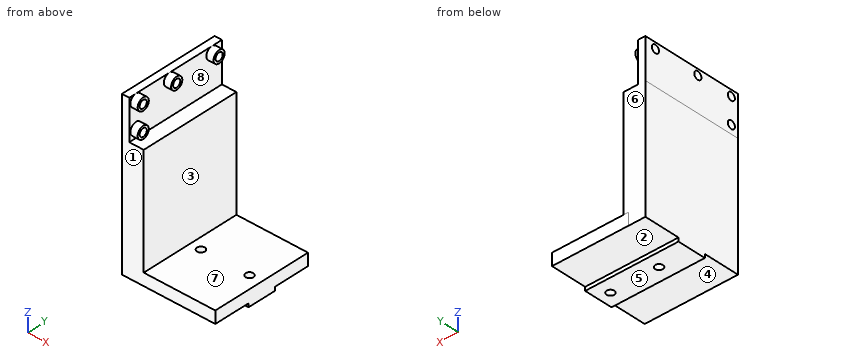
```python
from build123d import *

# Parameters (mm, degrees)
SKETCH1_W               = 31.5
SKETCH1_H               = 41.5
BOSS_EXTRUDE1_DEPTH     = 5
SKETCH3_W               = 6
SKETCH3_H               = 41.48411863
BOSS_EXTRUDE3_DEPTH     = 50.5
SKETCH5_W               = 3
SKETCH5_H               = 41.48411863
BOSS_EXTRUDE4_DEPTH     = 16.5
SKETCH6_W               = 50.5
SKETCH6_H               = 41.48411863
BOSS_EXTRUDE6_DEPTH     = 2
SKETCH4_R               = 2.5
SKETCH4_R_2             = 1.6
BOSS_EXTRUDE7_DEPTH     = 3
SKETCH4_6_R             = 1.6
CUT_EXTRUDE1_DEPTH      = 4
CUT_EXTRUDE1_DEPTH_BACK = 36.459931403
SKETCH7_W               = 1.5
SKETCH7_H               = 11.8
BOSS_EXTRUDE8_DEPTH     = 37.5
SKETCH8_R               = 1.6
CUT_EXTRUDE2_DEPTH      = 7.5
BOSS_EXTRUDE9_DEPTH     = 0.959931


with BuildPart() as part:
    # Sketch1 → Boss-Extrude1 (new body)
    with BuildSketch(Plane.XY):
        with Locations((-107.290068597, -86.48411863)):
            Rectangle(SKETCH1_W, SKETCH1_H)
    extrude(amount=BOSS_EXTRUDE1_DEPTH)

    # Sketch3 → Boss-Extrude3 (add)
    with BuildSketch(Plane.XY):
        with Locations((-126.040068597, -86.492059315)):
            Rectangle(SKETCH3_W, SKETCH3_H)
    extrude(amount=BOSS_EXTRUDE3_DEPTH)

    # Sketch5 → Boss-Extrude4 (add)
    with BuildSketch(Plane.XY.offset(50.5)):
        with Locations((-128.5, -86.492059315)):
            Rectangle(SKETCH5_W, SKETCH5_H)
    extrude(amount=BOSS_EXTRUDE4_DEPTH)

    # Sketch6 → Boss-Extrude6 (add)
    with BuildSketch(Plane(origin=(-123.040068597, 0, 0), x_dir=(0, 0, -1), z_dir=(1, 0, 0))):
        with Locations((-25.25, -86.492059315)):
            Rectangle(SKETCH6_W, SKETCH6_H)
    extrude(amount=BOSS_EXTRUDE6_DEPTH)

    # Sketch4 → Boss-Extrude7 (add)
    with BuildSketch(Plane.ZY.offset(127)):
        with Locations((54, -104.25)):
            Circle(SKETCH4_R)
        with Locations((54, -104.25)):
            Circle(SKETCH4_R_2, mode=Mode.SUBTRACT)
        with Locations((64.5, -104.25)):
            Circle(SKETCH4_R)
        with Locations((64.5, -104.25)):
            Circle(SKETCH4_R_2, mode=Mode.SUBTRACT)
        with Locations((64.5, -89.25)):
            Circle(SKETCH4_R)
        with Locations((64.5, -89.25)):
            Circle(SKETCH4_R_2, mode=Mode.SUBTRACT)
        with Locations((64.5, -70.25)):
            Circle(SKETCH4_R)
        with Locations((64.5, -70.25)):
            Circle(SKETCH4_R_2, mode=Mode.SUBTRACT)
    extrude(amount=-BOSS_EXTRUDE7_DEPTH)

    # Sketch4<6> → Cut-Extrude1 (cut, two sides)
    with BuildSketch(Plane.ZY.offset(127)) as cut_extrude1_sk:
        with Locations((64.5, -104.25)):
            Circle(SKETCH4_6_R)
        with Locations((64.5, -89.25)):
            Circle(SKETCH4_6_R)
        with Locations((64.5, -70.25)):
            Circle(SKETCH4_6_R)
        with Locations((54, -104.25)):
            Circle(SKETCH4_6_R)
    extrude(amount=CUT_EXTRUDE1_DEPTH, mode=Mode.SUBTRACT)
    extrude(cut_extrude1_sk.sketch, amount=-CUT_EXTRUDE1_DEPTH_BACK, mode=Mode.SUBTRACT)

    # Sketch7 → Boss-Extrude8 (add)
    with BuildSketch(Plane(origin=(-91.540068597, 0, 0), x_dir=(0, 0, -1), z_dir=(1, 0, 0))):
        with Locations((0.75, -86.48411863)):
            Rectangle(SKETCH7_W, SKETCH7_H)
    extrude(amount=-BOSS_EXTRUDE8_DEPTH)

    # Sketch8 → Cut-Extrude2 (cut, through all)
    with BuildSketch(Plane.XY.offset(5)):
        with Locations((-116.540068597, -86.490848024)):
            Circle(SKETCH8_R)
        with Locations((-96.540068597, -86.485464509)):
            Circle(SKETCH8_R)
    extrude(amount=-CUT_EXTRUDE2_DEPTH, mode=Mode.SUBTRACT)

    # Sketch9 → Boss-Extrude9 (add)
    with BuildSketch(Plane.ZY.offset(129.040068597)):
        Polygon((50.5, -65.75), (0, -65.75), (0, -80.58411863), (-1.5, -80.58411863), (-1.5, -92.38411863), (0, -92.38411863), (0, -107.23411863), (50.5, -107.23411863), align=None)
    extrude(amount=BOSS_EXTRUDE9_DEPTH)


solid = part.part
```
Check sheet for the modelled part. Datum: model origin and axes. Units: mm. Face numbers are marked on the shaded views. A direction names the side the tool comes from. Coordinates: 2 decimals unless noted, no trailing zeros. Loops run counter-clockwise (first coordinate to the right, second up) from the corner with the lowest first, then second, coordinate; pieces in that order, holes last. Notation, with made-up numbers: M 32,-7 L 78,-7 A12 ccw 78,14 Z; hole C 71.25,78.25 d9. An arc over 180 degrees is marked long. Answer as a JSON object with one key per item and string values.
1. Scan lines: L1, parallel to Z at x = -128.45, y = -104.25; L2, parallel to Z at x = -113, y = -97.5; L3, parallel to X at y = -69.5, z = 29.5. Record each from-to range of solid material in increasing order. Write a range as from..to.
Outcome:
{"L1": "0..52.4, 55.6..62.9, 66.1..67", "L2": "0..5", "L3": "-130..-121.04"}
2. Sectioned sample at C-C on z = 54. Record the cut outline in (x, y).
Outcome:
{"outline": "M -130,-107.23 L -127,-107.23 L -127,-106.75 L -124,-106.75 L -124,-105.85 L -130,-105.85 Z; M -130,-102.65 L -124,-102.65 L -124,-101.75 L -127,-101.75 L -127,-65.75 L -130,-65.75 Z"}
3. Sectioned sample at B-B on z = 64.5. Record the cut outline in (x, y), and give its area (3 significant figures).
Outcome:
{"outline": "M -130,-107.23 L -127,-107.23 L -127,-106.75 L -124,-106.75 L -124,-105.85 L -130,-105.85 Z; M -130,-102.65 L -124,-102.65 L -124,-101.75 L -127,-101.75 L -127,-91.75 L -124,-91.75 L -124,-90.85 L -130,-90.85 Z; M -130,-87.65 L -124,-87.65 L -124,-86.75 L -127,-86.75 L -127,-72.75 L -124,-72.75 L -124,-71.85 L -130,-71.85 Z; M -130,-68.65 L -124,-68.65 L -124,-67.75 L -127,-67.75 L -127,-65.75 L -130,-65.75 Z", "area": "112 mm²"}
4. Access from +Z, -Z, +X, -X, +Y, -Y to the whole of each face (thin tool, end or side, straight path). Record for the marked faces 1, 2, 3 and 4.
Outcome:
{"face 1": "+Z, -Z, +X, -X, -Y", "face 2": "-Z, +X, -X, +Y", "face 3": "+Z, +X, +Y, -Y", "face 4": "-Z, +X, -X, -Y"}
5. Release check for a two-part mould opening along Z. For the marked faces 5, 6, 7 and 8 record: pulls with the +Z half, pulls with the -Z half, needs draft (parallel to the pull), parting line crosses it, or undercut.
Outcome:
{"face 5": "pulls with the -Z half", "face 6": "needs draft", "face 7": "pulls with the +Z half", "face 8": "undercut"}
6. Sectioned sample at D-D on y = -90. Record the cut outline in (x, z), and give its area (3 significant figures).
Outcome:
{"outline": "M -130,-1.5 L -91.54,-1.5 L -91.54,5 L -121.04,5 L -121.04,50.5 L -127,50.5 L -127,62.12 L -124,62.12 L -124,63.09 L -130,63.09 Z; M -130,65.91 L -124,65.91 L -124,66.88 L -127,66.88 L -127,67 L -130,67 Z", "area": "705 mm²"}
7. Sectioned sample at A-A on x = -125.5. Count the separate pieces of the cut face and the enclosed holes in it, and give its area (3 significant figures).
Outcome:
{"separate pieces": "5", "enclosed holes": "4", "area": "2,160 mm²"}
8. Depth check by flat-ended pin: P1, Ø1.8, axis at x = -123, y = -91, coming from the +Z side; P2, Ø12, axis at x = -98.5, y = -82.5, coming from the +Z side; P3, Ø18, axis at y = -87, z = 60.5, coming from the +X side; P4, Ø1.9, axis at y = -89.25, z = 64.5, coming from the +X side. Enter the tip coordinate at first touch or a pass-through.
Outcome:
{"P1": "z = 50.5", "P2": "z = 5", "P3": "x = -124", "P4": "through"}
